Input: part model. Units: mm. Frame: model coordinates. A direction names the side the tool comes from. Coordinates: 2 decimals unless noted, no trailing zeros. Loops run counter-clockwise (first coordinate to the right, second up) from the corner with the lowest first, then second, coordinate; pieces in that order, holes last. Notation, with made-up numbers: (16, 49) -> (54, 49) arc R23 cw to (54, 81) -> close; hole circle Ø9 at (58.5, 19.25). An arc over 180 degrees is marked (long way). Put each result on its own line as item: value. Start each with the question number.
1) Material intervals for L1, parallel to Z at x = -2, y = 23; L2, parallel to X at y = 7, z = -0.5; L3, parallel to Y at x = 0.5, z = 63.5, sorted ascending.
2) Pull-direction query (X, two-part tool) for faces 5 (the flat face through (0, 0, 90)), 6 (the cylindrical face through (-4.769, -21.477, 0.224)), 7 (the cylindrical face through (-13.962, -13.591, 65.042)); classes: pulls with the +X half, pulls with the -X half, needs draft (parallel to the pull), parting line crosses it, or undercut.
3) Set-up query: faces 1 (the flat face through (0, 40.062, -62)), 2 (the cylindrical face through (-20.03, 6.31, -31.78)), 3 (the flat face through (12, -12, 62)), 4 (the flat face through (0, 3, 84)). Return all of +Z, -Z, +X, -X, +Y, -Y with unobstructed straight access to the full face (end or side cutting, diameter ignored); none if empty.
4) Contact query for flat-ended pins moving along their axis: P1, Ø1.5, axis at x = 17.5, y = 16.5, coming from the -Z side; P2, Ø12, axis at x = -1, z = -7.5, coming from the +Y side; P3, Ø1, axis at y = 20.5, z = -5.5, coming from the -X side; P4, Ø14, axis at y = 28, z = -67, coming from the -X side. Output: stop coordinate, or through.
5) Cut plane A-A (z = -51). Return the cut outline in (x, y).
6) Cut plane D-D (z = 64). Return the cut outline in (x, y).
7) Cut plane B-B (y = 0). Return the cut outline in (x, z), plus the area to 3 significant figures.
from build123d import *

# Parameters (mm, degrees)
SKETCH1_R                = 22
BOSS_EXTRUDE1_DEPTH      = 16
BOSS_EXTRUDE1_DEPTH_BACK = 16
SKETCH2_R                = 20.85
BOSS_EXTRUDE2_DEPTH      = 8
SKETCH3_R                = 20.85
BOSS_EXTRUDE3_DEPTH      = 44
SKETCH4_R                = 21
BOSS_EXTRUDE4_DEPTH      = 32
SKETCH5_R                = 23.25
BOSS_EXTRUDE5_DEPTH      = 28.5
BOSS_EXTRUDE6_DEPTH      = 28.5
SKETCH7_R                = 12
BOSS_EXTRUDE7_DEPTH      = 2
SKETCH8_R                = 2
CUT_EXTRUDE1_DEPTH       = 6
SKETCH9_W                = 24.120250452
SKETCH9_H                = 20.982117735
BOSS_EXTRUDE8_DEPTH      = 2
SKETCH10_R               = 4
BOSS_EXTRUDE9_DEPTH      = 20
CUT_EXTRUDE2_DEPTH       = 12


with BuildPart() as part:
    # Sketch1 → Boss-Extrude1 (new body, two sides)
    with BuildSketch(Plane.XY) as boss_extrude1_sk:
        Circle(SKETCH1_R)
    extrude(amount=BOSS_EXTRUDE1_DEPTH)
    extrude(boss_extrude1_sk.sketch, amount=-BOSS_EXTRUDE1_DEPTH_BACK)

    # Sketch2 → Boss-Extrude2 (add)
    with BuildSketch(Plane.XY.offset(16)):
        Circle(SKETCH2_R)
    extrude(amount=BOSS_EXTRUDE2_DEPTH)

    # Sketch3 → Boss-Extrude3 (add)
    with BuildSketch(Plane.XY.offset(24)):
        Circle(SKETCH3_R)
    extrude(amount=BOSS_EXTRUDE3_DEPTH)

    # Sketch4 → Boss-Extrude4 (add)
    with BuildSketch(Plane(origin=(0, 0, -16), x_dir=(-1, 0, 0), z_dir=(0, 0, -1))):
        Circle(SKETCH4_R)
    extrude(amount=BOSS_EXTRUDE4_DEPTH)

    # Sketch5 → Boss-Extrude5 (add)
    with BuildSketch(Plane(origin=(0, 0, -48), x_dir=(-1, 0, 0), z_dir=(0, 0, -1))):
        Circle(SKETCH5_R)
    extrude(amount=BOSS_EXTRUDE5_DEPTH)

    # Sketch6 → Boss-Extrude6 (add)
    with BuildSketch(Plane(origin=(0, 0, -76.5), x_dir=(-1, 0, 0), z_dir=(0, 0, -1))):
        with BuildLine():
            Line((14, 40.062394781), (-14, 40.062394781))
            Line((-14, 40.062394781), (-14, 18.562394781))
            ThreePointArc((-14, 18.562394781), (-12.776481168, 19.424830217), (-11.5, 20.206743924))
            Line((-11.5, 20.206743924), (-11.5, 37.562394781))
            Line((-11.5, 37.562394781), (11.5, 37.562394781))
            Line((11.5, 37.562394781), (11.5, 20.206743924))
            ThreePointArc((11.5, 20.206743924), (12.776481168, 19.424830217), (14, 18.562394781))
            Line((14, 18.562394781), (14, 40.062394781))
        make_face()
    extrude(amount=-BOSS_EXTRUDE6_DEPTH)

    # Sketch7 → Boss-Extrude7 (add)
    with BuildSketch(Plane.XY.offset(68)):
        Circle(SKETCH7_R)
    extrude(amount=BOSS_EXTRUDE7_DEPTH)

    # Sketch8 → Cut-Extrude1 (cut)
    with BuildSketch(Plane.XY.offset(68)):
        with Locations((12.374368671, 12.374368671)):
            Circle(SKETCH8_R)
        with Locations((12.374368671, -12.374368671)):
            Circle(SKETCH8_R)
        with Locations((-12.374368671, -12.374368671)):
            Circle(SKETCH8_R)
        with Locations((-12.374368671, 12.374368671)):
            Circle(SKETCH8_R)
    extrude(amount=-CUT_EXTRUDE1_DEPTH, mode=Mode.SUBTRACT)

    # Sketch9 → Boss-Extrude8 (add)
    with BuildSketch(Plane(origin=(0, 0, -76.5), x_dir=(-1, 0, 0), z_dir=(0, 0, -1))):
        with Locations((0, 27.637719743)):
            Rectangle(SKETCH9_W, SKETCH9_H)
    extrude(amount=-BOSS_EXTRUDE8_DEPTH)

    # Sketch10 → Boss-Extrude9 (add)
    with BuildSketch(Plane.XY.offset(70)):
        Circle(SKETCH10_R)
    extrude(amount=BOSS_EXTRUDE9_DEPTH)

    # Sketch11 → Cut-Extrude2 (cut)
    with BuildSketch(Plane.XY.offset(90)):
        Polygon((0, 3), (-3.981730615, 3), (-3.981730615, 4.192756348), (4.050863087, 4.192756348), (4.050863087, 3), align=None)
    extrude(amount=-CUT_EXTRUDE2_DEPTH, mode=Mode.SUBTRACT)


solid = part.part
Results found:
1. L1: z = -76.5 to -48
1. L2: x = -20.86 to 20.86
1. L3: y = -20.84 to 20.84
2. face 5: needs draft
2. face 6: parting line crosses it
2. face 7: undercut
3. face 1: +Z, -Z, +X, -X, +Y
3. face 2: none
3. face 3: +Z
3. face 4: +Z, +X, -X, +Y
4. P1: passes through
4. P2: stops at y = 22
4. P3: stops at x = -9.17
4. P4: stops at x = -14
5. outline: (-14, 18.56) arc R23.25 ccw (long way) to (14, 18.56) -> (14, 40.06) -> (-14, 40.06) -> close; hole (-11.5, 20.21) arc R23.25 cw to (11.5, 20.21) -> (11.5, 37.56) -> (-11.5, 37.56) -> close
6. outline: circle Ø41.7 at (0, 0); hole circle Ø4 at (-12.37, -12.37); hole circle Ø4 at (-12.37, 12.37); hole circle Ø4 at (12.37, -12.37); hole circle Ø4 at (12.37, 12.37)
7. outline: (-23.25, -76.5) -> (23.25, -76.5) -> (23.25, -48) -> (21, -48) -> (21, -16) -> (22, -16) -> (22, 16) -> (20.85, 16) -> (20.85, 68) -> (12, 68) -> (12, 70) -> (4, 70) -> (4, 90) -> (-4, 90) -> (-4, 70) -> (-12, 70) -> (-12, 68) -> (-20.85, 68) -> (-20.85, 16) -> (-22, 16) -> (-22, -16) -> (-21, -16) -> (-21, -48) -> (-23.25, -48) -> close
7. area: 6,450 mm2
